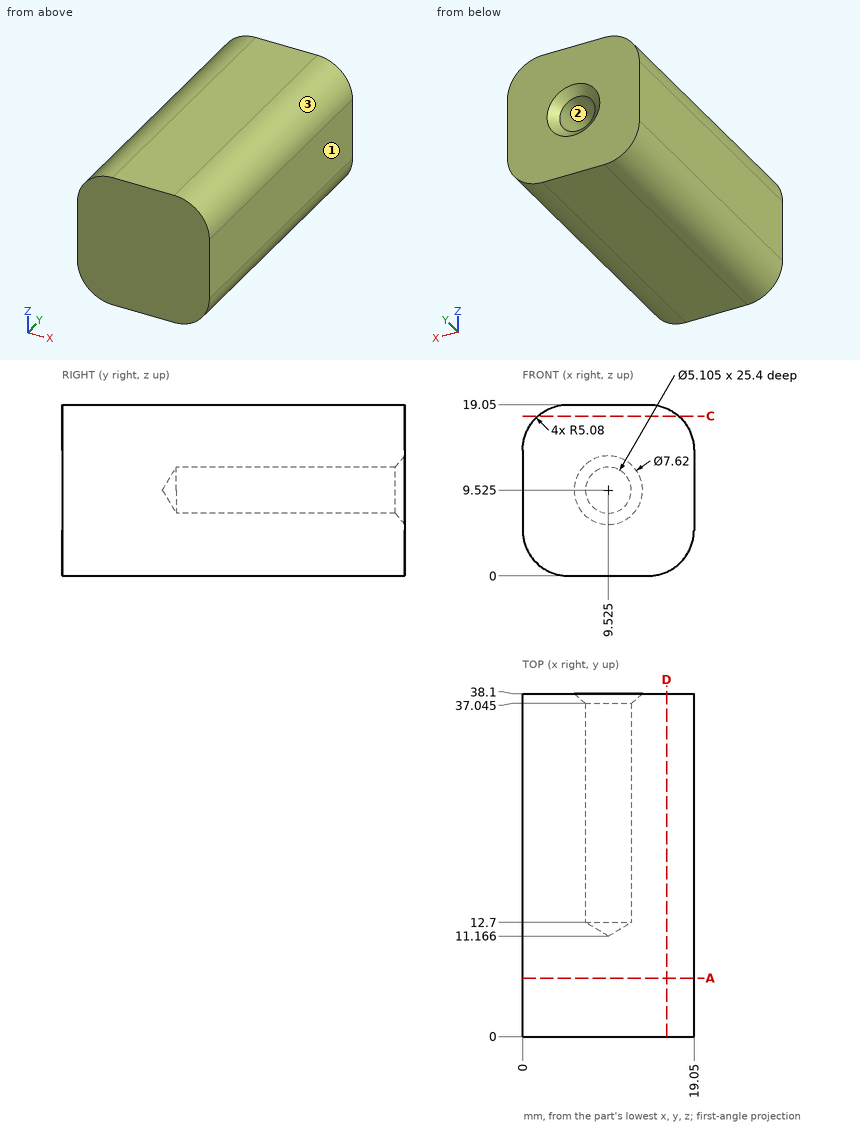
Design review of the part shown in the three views and the two pictorial views. Dimensions are in mm from the part's minimum x, y and z. Round coordinates to 2 decimals unless told otherwise and drop trailing zeros. Order: outer loops, then holes, each group sorted by start corner. A loop starts at its lowest first (then second) coordinate and runs counter-clockwise, first axis right, second up. Notation, with made-up numbers: (24, 65) - (28, 65) arc R18 cw to (28, 90) - close; hole circle Ø1 at (26.5, 54.25). An arc over 180 degrees is marked (long way). Answer in a Markdown table with one row per item.
(1) Take a section at C-C on z = 17.75. Write out the cut boundary in (x, y).
Result set:
| item | result |
|---|---|
| outline | (1.69, 0) - (17.36, 0) - (17.36, 38.1) - (1.69, 38.1) - close |
(2) For line 1 (X direction, y = 26.5, z = 9.5); line 2 (Z direction, x = 17, y = 28), list the stretches that pass through material, from the lowest coordinate up. Write a range as from..to.
Result set:
| item | result |
|---|---|
| line 1 | x = 0..6.97, 12.08..19.05 |
| line 2 | z = 1..18.05 |
(3) Mouldability with a two-part tool opening along Z and no side actions: class the marked faces 1, 2 and 3 as released by +Z, released by -Z, zero draft, split by the parting line, or undercut.
Result set:
| item | result |
|---|---|
| face 1 | zero draft |
| face 2 | undercut |
| face 3 | released by +Z |
(4) Take a section at A-A on y = 6.5. Write out the cut boundary in (x, z), plus the area to 3 significant figures.
Result set:
| item | result |
|---|---|
| outline | (0, 5.08) arc R5.08 ccw to (5.08, 0) - (13.97, 0) arc R5.08 ccw to (19.05, 5.08) - (19.05, 13.97) arc R5.08 ccw to (13.97, 19.05) - (5.08, 19.05) arc R5.08 ccw to (0, 13.97) - close |
| area | 341 mm2 |
(5) Take a section at D-D on x = 16. Write out the cut boundary in (y, z).
Result set:
| item | result |
|---|---|
| outline | (0, 0.42) - (38.1, 0.42) - (38.1, 18.63) - (0, 18.63) - close |
